from build123d import *

# Parameters (mm, degrees)
BOSS_EXTRUDE1_DEPTH           = 6.35
CSK_FOR_M4_SFHCS1_D           = 4.5
CSK_FOR_M4_SFHCS1_CSINK_D     = 8.96
CSK_FOR_M4_SFHCS1_CSINK_ANGLE = 90


with BuildPart() as part:
    # Sketch1 → Boss-Extrude1 (new body)
    with BuildSketch(Plane(origin=(0, 0, 0), x_dir=(1, 0, 0), z_dir=(0, 1, 0))):
        with BuildLine():
            Line((230.928932188, -255), (-230.928932188, -255))
            ThreePointArc((-230.928932188, -255), (-232.84234935, -255.380602337), (-234.464466094, -256.464466094))
            Line((-234.464466094, -256.464466094), (-246.535533906, -268.535533906))
            ThreePointArc((-246.535533906, -268.535533906), (-248.15765065, -269.619397663), (-250.071067812, -270))
            Line((-250.071067812, -270), (-253, -270))
            ThreePointArc((-253, -270), (-256.535533906, -268.535533906), (-258, -265))
            Line((-258, -265), (-258, 262.5))
            ThreePointArc((-258, 262.5), (-257.267766953, 264.267766953), (-255.5, 265))
            Line((-255.5, 265), (-250.5, 265))
            ThreePointArc((-250.5, 265), (-248.732233047, 264.267766953), (-248, 262.5))
            Line((-248, 262.5), (-248, 260))
            ThreePointArc((-248, 260), (-246.535533906, 256.464466094), (-243, 255))
            Line((-243, 255), (-18, 255))
            ThreePointArc((-18, 255), (-10.928932188, 257.928932188), (-8, 265))
            Line((-8, 265), (-8, 270))
            ThreePointArc((-8, 270), (-6.535533906, 273.535533906), (-3, 275))
            Line((-3, 275), (3, 275))
            ThreePointArc((3, 275), (6.535533906, 273.535533906), (8, 270))
            Line((8, 270), (8, 265))
            ThreePointArc((8, 265), (10.928932188, 257.928932188), (18, 255))
            Line((18, 255), (243, 255))
            ThreePointArc((243, 255), (246.535533906, 256.464466094), (248, 260))
            Line((248, 260), (248, 262.5))
            ThreePointArc((248, 262.5), (248.732233047, 264.267766953), (250.5, 265))
            Line((250.5, 265), (255.5, 265))
            ThreePointArc((255.5, 265), (257.267766953, 264.267766953), (258, 262.5))
            Line((258, 262.5), (258, -265))
            ThreePointArc((258, -265), (256.535533906, -268.535533906), (253, -270))
            Line((253, -270), (250.071067812, -270))
            ThreePointArc((250.071067812, -270), (248.15765065, -269.619397663), (246.535533906, -268.535533906))
            Line((246.535533906, -268.535533906), (234.464466094, -256.464466094))
            ThreePointArc((234.464466094, -256.464466094), (232.84234935, -255.380602337), (230.928932188, -255))
        make_face()
    extrude(amount=BOSS_EXTRUDE1_DEPTH)

    # CSK for M4 SFHCS1 (through all)
    with Locations(Plane(origin=(0, 6.35, 0), x_dir=(1, 0, 0), z_dir=(0, 1, 0))):
        with Locations((0, 270), (253, -265), (-253, -265)):
            CounterSinkHole(CSK_FOR_M4_SFHCS1_D / 2, CSK_FOR_M4_SFHCS1_CSINK_D / 2, counter_sink_angle=CSK_FOR_M4_SFHCS1_CSINK_ANGLE)


solid = part.part
Work out the finished part from the listing and answer in its coordinate system (mm). A direction names the side the tool comes from. Give positions to 0.01 mm unless a question says otherwise; leave off trailing zeros. Order: outer loops, then holes, each group sorted by start corner. A loop starts at its lowest first (then second) coordinate and runs counter-clockwise, first axis right, second up. Notation, with made-up numbers: (16, 61.25) - (56, 61.25) arc R21 ccw to (56, 98.25) - close; hole circle Ø3 at (12.25, 19.5). An arc over 180 degrees is marked (long way). Answer as CSV lines item,"result". Start each with the question number.
Q1. For faces 1 (the face through (241, 3, 263)), 2 (the face through (4, 0, -6)), determine the directions among +Z, -Z, +X, -X, +Y, -Y from which every point of the face is accessible in a straight line to the end or side of a thin tool.
Q2. Find the intervals of material crossed by L1, parallel to X at y = 1.6, z = 265; L2, parallel to Z at x = 253, y = 2.9; L3, parallel to Z at x = 0, y = 3.1, in increasing order. Write a range as [from, to].
Q3. Given pin 1 Ø6 at (x, z) = (-253, 265) entering from -Y; pin 2 Ø3 at (x, y) = (108.5, 4.5) entering from -Z; pin 3 Ø3 at (x, y) = (-62.5, 5.5) entering from +Z; pin 4 Ø6 at (x, z) = (0, -270) entering from +Y, each flat-ended and moving along its own axis, determine where each tip first touches the part or whether it passes through.
Q4. The part is cut by section A-A (y = 2.75). Give the number of separate pieces and of enclosed holes in the cut face, then the cut area to 3 significant figures.
Q5. The mould has two halves that part along X. Classify faces 3 (the face through (-240, 3, 262)), 4 (the face through (4, 6.35, -6)): +X half, -X half, draft (parallel to the pull), parting line (faces both ways), or undercut.
Q6. The part is cut by section B-B (x = -147). Write down the section's boundary in (y, z).
Check result:
1,face 1,"+Z, +Y, -Y"
1,face 2,"+Z, -Z, +X, -X, -Y"
2,L1,"x = [-258, -255.25], [-250.75, -243], [243, 250.75], [255.25, 258]"
2,L2,"z = [-265, 262.75], [267.25, 270]"
2,L3,"z = [-275, -272.25], [-267.75, 255]"
3,pin 1,"stops at y = 0"
3,pin 2,"stops at z = -255"
3,pin 3,"stops at z = 255"
3,pin 4,"stops at y = 4.87"
4,separate pieces,"1"
4,enclosed holes,"3"
4,area,"264,000 mm²"
5,face 3,"undercut"
5,face 4,"draft"
6,outline,"(0, -255) - (6.35, -255) - (6.35, 255) - (0, 255) - close"
